Geometry check sheet. Reference: drawing and pictorial views, mm from the part's lowest x, y, z. A direction names the side the tool comes from. Give positions to 0.01 mm unless a question says otherwise; leave off trailing zeros. Write each loop counter-clockwise with the first axis right and the second up, starting at its lowest first coordinate (ties: lowest second). Pieces come first, ordered by that corner, then holes. Notation, with made-up numbers: (1, 30.25) - (50, 30.25) arc R25 cw to (50, 68.25) - close; hole circle Ø9 at (73, 17). An arc over 180 degrees is marked (long way). Put each result on its own line as item: value.
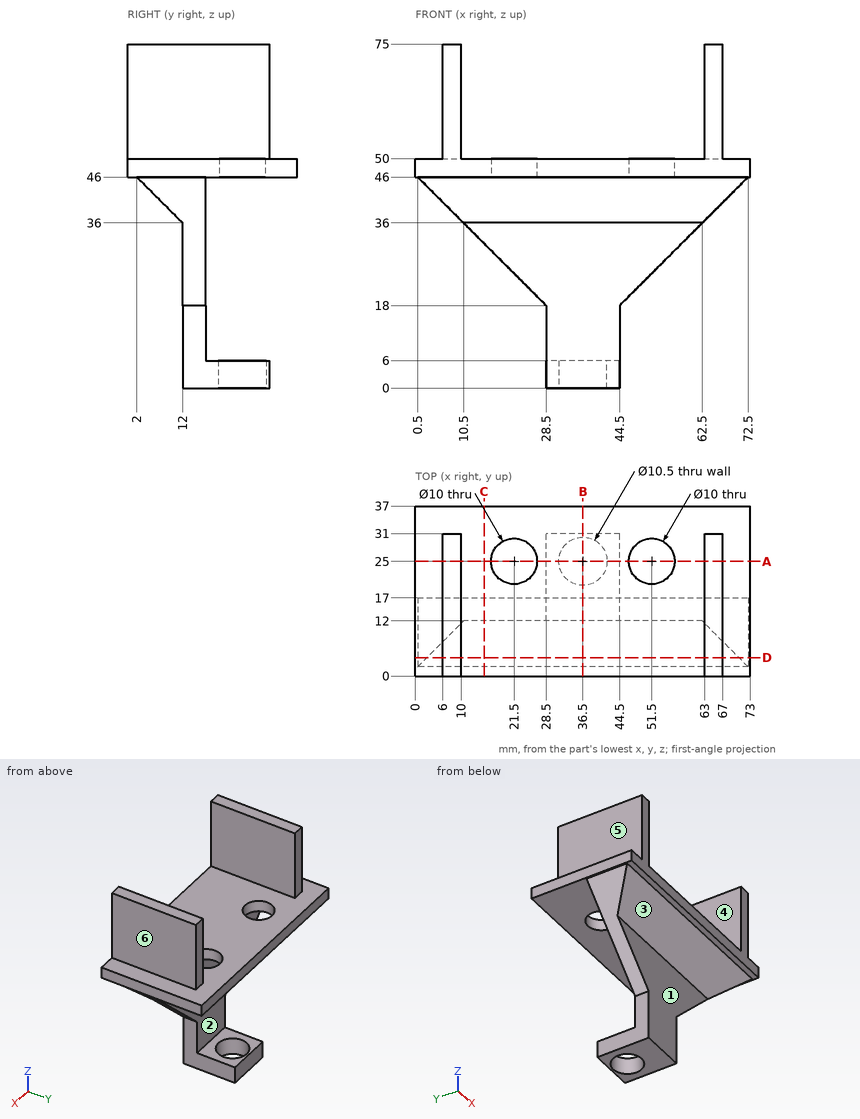
Q1. Section check C-C, the plane x = 15. Record the cut outline in (y, z), plus the area to 4 significant figures.
Answers follow:
outline: (0, 46) - (2, 46) - (12, 36) - (12, 31.5) - (17, 31.5) - (17, 46) - (37, 46) - (37, 50) - (0, 50) - close
area: 270.5 mm2
Q2. Section check B-B, the plane x = 36.5. Record the cut outline in (y, z).
Answers follow:
outline: (0, 46) - (2, 46) - (12, 36) - (12, 0) - (19.75, 0) - (19.75, 6) - (17, 6) - (17, 46) - (37, 46) - (37, 50) - (0, 50) - close; (30.25, 0) - (31, 0) - (31, 6) - (30.25, 6) - close
Q3. Release check for a two-part mould opening along Z. For the marked faces 1, 2 and 3 record: released by +Z, released by -Z, zero draft, split by the parting line, or undercut.
Answers follow:
face 1: zero draft
face 2: undercut
face 3: released by -Z
Q4. Scan lines: line 1 along X through (y, z) = (25, 47.95); line 2 along X through (y, z) = (23, 61.5); line 3 along Y through (x, z) = (21.5, 47.7). Record each from-to range of solid material in increasing order.
Answers follow:
line 1: x = 0 to 16.5, 26.5 to 46.5, 56.5 to 73
line 2: x = 6 to 10, 63 to 67
line 3: y = 0 to 20, 30 to 37
Q5. Section check A-A, the plane y = 25. Record the cut outline in (x, z), plus the area to 3 significant figures.
Answers follow:
outline: (0, 46) - (16.5, 46) - (16.5, 50) - (10, 50) - (10, 75) - (6, 75) - (6, 50) - (0, 50) - close; (26.5, 46) - (46.5, 46) - (46.5, 50) - (26.5, 50) - close; (28.5, 0) - (31.25, 0) - (31.25, 6) - (28.5, 6) - close; (41.75, 0) - (44.5, 0) - (44.5, 6) - (41.75, 6) - close; (56.5, 46) - (73, 46) - (73, 50) - (67, 50) - (67, 75) - (63, 75) - (63, 50) - (56.5, 50) - close
area: 445 mm2
Q6. Go/stop test with flat-tipped pins: pin 1 Ø18.5 at (x, y) = (53, 17) entering from +Z; pin 2 Ø12.5 at (y, z) = (19, 65) entering from -X; pin 3 Ø1.2 at (x, z) = (7, 61) entering from +Y. Record where each tip stops, or that it passes through.
Answers follow:
pin 1: stops at z = 50
pin 2: stops at x = 6
pin 3: stops at y = 31
Q7. Set-up check for the marked faces 4, 5 and 6: record each of +Z, -Z, +X, -X, +Y, -Y from which the full face is reachable in a straight line by a thin tool's end or side.
Answers follow:
face 4: +Z, +Y, -Y
face 5: +Z, -X, +Y, -Y
face 6: +Z, +X, +Y, -Y
Q8. Section check D-D, the plane y = 4. Record the cut outline in (x, z), plus the area to 3 significant figures.
Answers follow:
outline: (0, 46) - (0.5, 46) - (2.5, 44) - (70.5, 44) - (72.5, 46) - (73, 46) - (73, 50) - (67, 50) - (67, 75) - (63, 75) - (63, 50) - (10, 50) - (10, 75) - (6, 75) - (6, 50) - (0, 50) - close
area: 632 mm2
